Autodesk Inventor part; units mm, degrees
ref_plane "YZ Plane" through (0, 0, 0) normal (1, 0, 0) x (0, 1, 0)
ref_plane "XZ Plane" through (0, 0, 0) normal (0, 1, 0) x (-1, 0, 0)
ref_plane "XY Plane" through (0, 0, 0) normal (0, 0, 1) x (1, 0, 0)
sketch "Sketch1" plane through (0, 0, 0) normal (0, 0, 1) x (1, 0, 0)
  line L0 (-92, -76) -> (92, -76)
  line L1 (92, -76) -> (92, 76)
  line L2 (92, 76) -> (-92, 76) construction
  line L3 (-92, 76) -> (-92, -76)
  line L4 (-92, -76) -> (92, 76) construction
  line L5 (92, -76) -> (-92, 76) construction
  line L6 (-92, -76) -> (-94, -76) construction
  line L7 (-92, 76) -> (-94, 76) construction
  line L8 (-92, -76) -> (-92, -78) construction
  line L9 (-94, 76) -> (-94, -78)
  line L10 (92, -76) -> (94, -76) construction
  line L11 (92, -76) -> (92, -78) construction
  line L12 (92, 76) -> (94, 76) construction
  line L13 (94, 76) -> (94, -78)
  line L14 (94, -78) -> (-94, -78)
  line L15 (-94, 76) -> (-92, 76)
  line L16 (92, 76) -> (94, 76)
  point P0 (0, 0)
  dimension "d0" = 184
  dimension "d1" = 152
  dimension "d2" = 2
  dimension "d3" = 2
  dimension "d4" = 2
  dimension "d5" = 2
  dimension "d6" = 2
  dimension "d7" = 2
  dimension "d8" = 2
extrude "Extrusion1" add sketch "Sketch1" along normal blind 80
sketch "Sketch2" plane through (0, 0, 80) normal (0, 0, 1) x (1, 0, 0)
  line L0 (92, -76) -> (-92, -76) construction
  line L1 (-92, -76) -> (-92, 76) construction
  line L2 (-92, 76) -> (-94, 76) construction
  line L3 (-94, 76) -> (-94, -78) construction
  line L4 (-94, -78) -> (94, -78) construction
  line L5 (94, -78) -> (94, 76) construction
  line L6 (94, 76) -> (92, 76) construction
  line L7 (92, 76) -> (92, -76) construction
  line L8 (-94, -78) -> (-94, 76)
  line L9 (94, -78) -> (94, 76)
  line L10 (-94, 76) -> (94, 76)
  line L11 (94, 76) -> (94, -78)
  line L12 (94, -78) -> (-94, -78)
  line L13 (-94, -78) -> (-94, 76)
  point P0 (0, 0)
extrude "Extrusion2" add sketch "Sketch2" along normal blind 2
sketch "Sketch3" plane through (-94, -78, 0) normal (-1, 0, 0) x (0, 0, 1)
  line L0 (0, 0) -> (0, 154) construction
  line L1 (0, 0) -> (82, 0) construction
  line L2 (82, 154) -> (82, 0) construction
  line L3 (0, 154) -> (82, 154) construction
  line L4 (0, 154) -> (80, 154) construction
  line L5 (0, 0) -> (2, 0)
  line L6 (2, 0) -> (2, 154)
  line L7 (2, 154) -> (0, 154)
  line L8 (0, 154) -> (0, 0)
  point P0 (0, 78)
  dimension "d13" = 2
extrude "Extrusion3" add sketch "Sketch3" along normal blind 12
sketch "Sketch4" plane through (94, -78, 0) normal (1, 0, 0) x (0, 0, -1)
  line L0 (0, 154) -> (0, 0) construction
  line L1 (0, 154) -> (-82, 154) construction
  line L2 (-82, 0) -> (-82, 154) construction
  line L3 (0, 0) -> (-82, 0) construction
  line L4 (0, 154) -> (0, 2)
  line L5 (-2, 0) -> (-82, 0) construction
  line L6 (0, 154) -> (-2, 154)
  line L7 (-2, 154) -> (-2, 0)
  line L8 (-2, 0) -> (0, 0)
  line L9 (0, 0) -> (0, 154)
  point P0 (0, 78)
extrude "Extrusion4" add sketch "Sketch4" along normal blind 12
sketch "Sketch5" plane through (-94, -78, 2) normal (0, 0, 1) x (1, 0, 0)
  circle A0 centre (-6, 15) radius 3 construction
  line L0 (0, 154) -> (0, 0) construction
  line L1 (0, 154) -> (-12, 154) construction
  line L2 (-12, 0) -> (-12, 154) construction
  line L3 (0, 0) -> (-12, 0) construction
  circle A1 centre (-6, 140) radius 3 construction
  line L4 (188, 154) -> (0, 154) construction
  line L5 (0, 154) -> (0, 0) construction
  line L6 (0, 0) -> (188, 0) construction
  line L7 (188, 0) -> (188, 154) construction
  line L8 (188, 154) -> (0, 154) construction
  line L9 (94, 154) -> (94, 2) construction
  line L10 (2, 2) -> (186, 2) construction
  circle A2 centre (194, 15) radius 3 construction
  circle A3 centre (194, 140) radius 3 construction
  point P0 (94, 78)
  dimension "d18" = 6
  dimension "d19" = 15
  dimension "d23" = 6
  dimension "d24" = 125
  dimension "d25" = 100
hole "Hole1" at (-100, 62, 2) at (-100, -63, 2) at (100, -63, 2) at (100, 62, 2) direction (0, 0, -1) diameter 6 end through all
fillet "Fillet1" radius 2 9 edges at (-106, 76, 1) (-106, -78, 1) (106, -78, 1) (106, 76, 1) (94, -1, 82) (-94, -1, 82) (-94, -78, 42) (94, -78, 42) (0, -78, 82)
fillet "Fillet1" radius 0.25 6 edges at (0, 76, 80) (92, 76, 40) (-92, 76, 40) (-94, 76, 42) (0, 76, 82) (94, 76, 42)
properties part number "BatteryBox_NP1812" material "Steel, Galvanized"
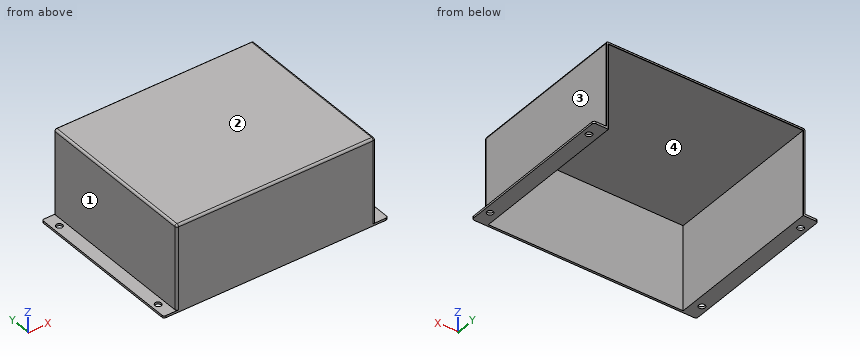
Here's how the part is built. I have some questions about the finished solid (model axes, mm). Face numbers are marked on the shaded views. A direction names the side the tool comes from. Round coordinates to 2 decimals unless told otherwise and drop trailing zeros. Order: outer loops, then holes, each group sorted by start corner. A loop starts at its lowest first (then second) coordinate and runs counter-clockwise, first axis right, second up. Notation, with made-up numbers: (63, 31) -> (81, 31) arc R17 cw to (81, 35) -> close; hole circle Ø9 at (82.5, 34.5). An arc over 180 degrees is marked (long way). Use CSV: the item, a comma, the result in double quotes.
1. I want a section at D-D on x = -43. List the corners of the cut face in (y, z) for me.
Recorded:
outline,"(-78, 0) -> (-76, 0) -> (-76, 80) -> (75.75, 80) arc R0.25 ccw to (76, 80.25) -> (76, 81.75) arc R0.25 ccw to (75.75, 82) -> (-76, 82) arc R2 ccw to (-78, 80) -> close"
2. I need wall thicknesses on line 1 along X through (y, z) = (62, 1.15); line 2 along Y through (x, z) = (100, 1.4); line 3 along X through (y, z) = (-46, 36.5). Which ranges of each line are inside material? Lowest first, please.
Recorded:
line 1,"x = -106 to -103, -97 to -92, 92 to 97, 103 to 106"
line 2,"y = -78 to -66, -60 to 59, 65 to 76"
line 3,"x = -94 to -92, 92 to 94"
3. I want a section at C-C on z = 5. List the corners of the cut face in (x, y) for me, and give its area (3 significant figures).
Recorded:
outline,"(-94, -76) arc R2 ccw to (-92, -78) -> (92, -78) arc R2 ccw to (94, -76) -> (94, 75.75) arc R0.25 ccw to (93.75, 76) -> (92.25, 76) arc R0.25 ccw to (92, 75.75) -> (92, -76) -> (-92, -76) -> (-92, 75.75) arc R0.25 ccw to (-92.25, 76) -> (-93.75, 76) arc R0.25 ccw to (-94, 75.75) -> close"
area,"982 mm2"
4. I want a section at A-A on y = -63. List the corners of the cut face in (x, z) for me, and give its area (3 significant figures).
Recorded:
outline,"(-106, 0) -> (-103, 0) -> (-103, 2) -> (-106, 2) -> close; (-97, 0) -> (-92, 0) -> (-92, 80) -> (92, 80) -> (92, 0) -> (97, 0) -> (97, 2) -> (94, 2) -> (94, 80) arc R2 ccw to (92, 82) -> (-92, 82) arc R2 ccw to (-94, 80) -> (-94, 2) -> (-97, 2) -> close; (103, 0) -> (106, 0) -> (106, 2) -> (103, 2) -> close"
area,"718 mm2"
5. I'm going to push flat-ended pins straight in: P1, Ø9.5, axis at x = 100, y = -63, coming from the +Z side; P2, Ø1.5, axis at x = 35.5, y = -49, coming from the -Z side; P3, Ø10, axis at y = 25, z = 71, coming from the -X side; P4, Ø3.5, axis at x = -100, y = 62, coming from the +Z side. Where does each tip first touch, or does it pass through?
Recorded:
P1,"stops at z = 2"
P2,"stops at z = 80"
P3,"stops at x = -94"
P4,"passes through"
6. I want a section at B-B on x = -100. List the corners of the cut face in (y, z) for me, and give its area (3 significant figures).
Recorded:
outline,"(-78, 0) -> (-66, 0) -> (-66, 2) -> (-78, 2) -> close; (-60, 0) -> (59, 0) -> (59, 2) -> (-60, 2) -> close; (65, 0) -> (76, 0) -> (76, 2) -> (65, 2) -> close"
area,"284 mm2"
7. Which directions (+Z, -Z, +X, -X, +Y, -Y) give clear straight access to the entire face, cutting with the end or side of a thin tool? Please do the marked faces 1, 2, 3 and 4.
Recorded:
face 1,"+Z, -X, +Y, -Y"
face 2,"+Z, +X, -X, +Y, -Y"
face 3,"+Z, +X, +Y, -Y"
face 4,"-Z, +Y"
